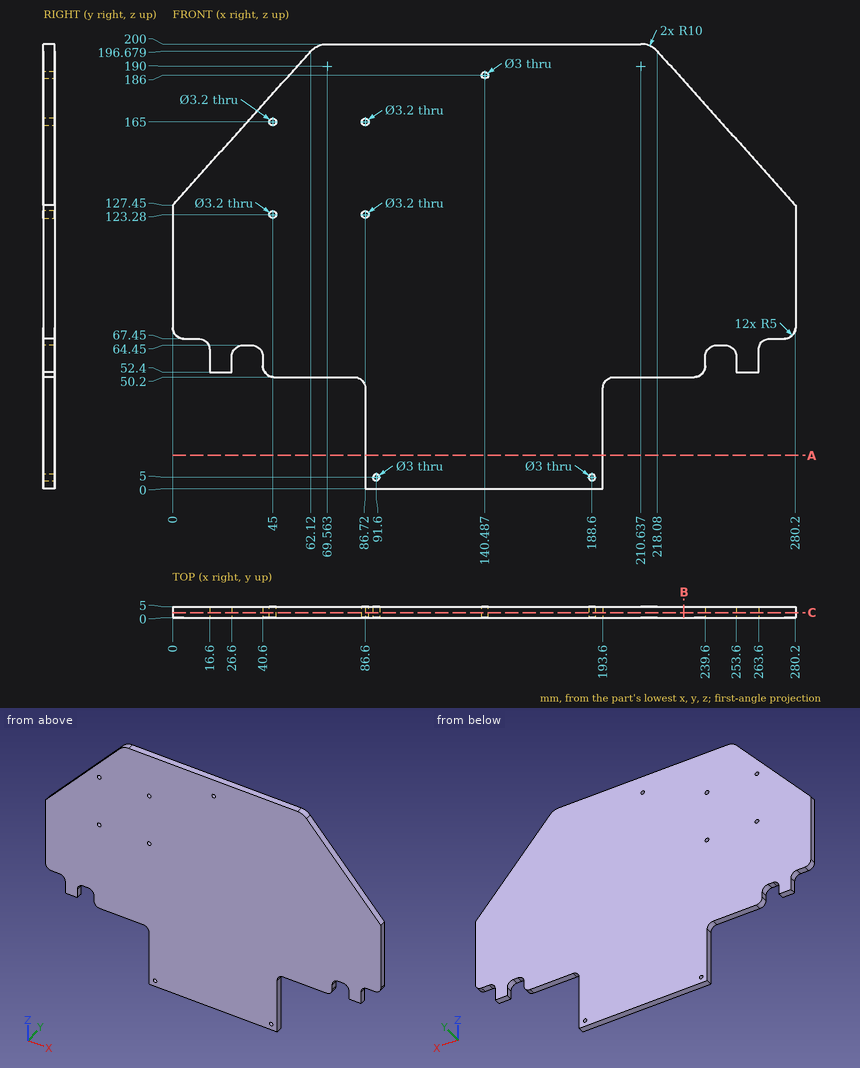
Can you work these out from the drawing? Everything is in mm from the part's minimum corner. Round coordinates to 2 decimals unless told otherwise and drop trailing zeros. Write each loop counter-clockwise with the first axis right and the second up, starting at its lowest first coordinate (ties: lowest second). Pieces come first, ordered by that corner, then holes.
1. Suppose I cut it at C-C (y = 2.3). State how many separate pieces and enclosed holes the cut face has, and give its area (3 significant figures).
2. Suppose I cut it at A-A (z = 15). List the corners of the cut face in (x, y) for me.
3. Will these pins go through, and if not, where does the flat tip stop? pin 1 Ø3.5 at (x, z) = (140.49, 186) entering from +Y; pin 2 Ø1.5 at (y, z) = (1, 143) entering from -X; pin 3 Ø2.5 at (x, y) = (19.5, 3) entering from -Z; pin 4 Ø2 at (x, y) = (53, 2.5) entering from -Z.
4. I need wall thicknesses on L1, parallel to X at y = 3.4, z = 5; L2, parallel to X at y = 1.65, z = 123.28; L3, parallel to X at y = 2.4, z = 186 (1 decimal). Which ranges of each line are inside material? Lowest first, please.
5. Suppose I cut it at B-B (x = 230). List the corners of the cut face in (y, z) for me (1 decimal), and give its area (3 significant figures).
Answer sheet:
1. separate pieces: 1
1. enclosed holes: 7
1. area: 41,600 mm2
2. outline: (86.6, 0) - (193.6, 0) - (193.6, 5) - (86.6, 5) - close
3. pin 1: stops at y = 5
3. pin 2: stops at x = 13.28
3. pin 3: stops at z = 52.4
3. pin 4: stops at z = 50.2
4. L1: x = 86.6 to 90.1, 93.1 to 187.1, 190.1 to 193.6
4. L2: x = 0 to 43.4, 46.6 to 85.12, 88.32 to 280.2
4. L3: x = 52.5 to 139, 142 to 227.7
5. outline: (0, 50.2) - (5, 50.2) - (5, 183.4) - (0, 183.4) - close
5. area: 666 mm2
